from build123d import *

# Parameters (mm, degrees)
SKETCH1_W           = 25.4
SKETCH1_H           = 25.4
SKETCH1_W_2         = 22.225
SKETCH1_H_2         = 22.225
BOSS_EXTRUDE1_DEPTH = 330.2
SKETCH2_R           = 4.365625
SKETCH2_R_2         = 2.38125
CUT_EXTRUDE1_DEPTH  = 25.4


with BuildPart() as part:
    # Sketch1 → Boss-Extrude1 (new body)
    with BuildSketch(Plane(origin=(0, 0, 0), x_dir=(1, 0, 0), z_dir=(0, 1, 0))):
        Rectangle(SKETCH1_W, SKETCH1_H)
        Rectangle(SKETCH1_W_2, SKETCH1_H_2, mode=Mode.SUBTRACT)
    extrude(amount=BOSS_EXTRUDE1_DEPTH)

    # Sketch2 → Cut-Extrude1 (cut)
    with BuildSketch(Plane.XY.offset(12.7)):
        with Locations((0, 25.4)):
            Circle(SKETCH2_R)
        with Locations((0, 50.8)):
            Circle(SKETCH2_R)
        with Locations((0, 317.5)):
            Circle(SKETCH2_R_2)
        with Locations((0, 114.3)):
            Circle(SKETCH2_R_2)
    extrude(amount=-CUT_EXTRUDE1_DEPTH, mode=Mode.SUBTRACT)


solid = part.part
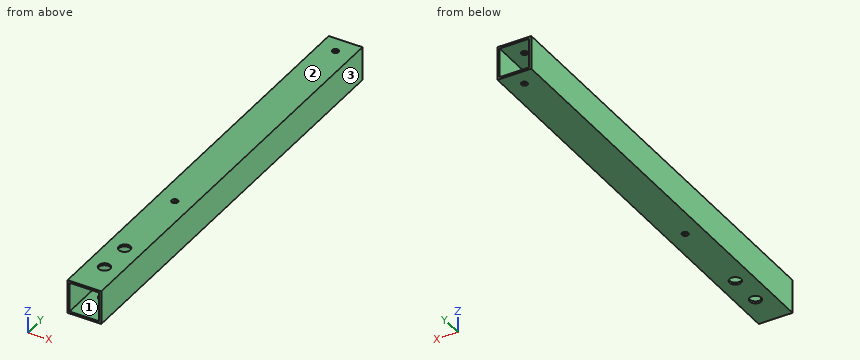
Verification items for the finished model (mm, model axes). Face numbers are marked on the shaded views. Give positions to 0.01 mm unless a question says otherwise; leave off trailing zeros. Loops run counter-clockwise (first coordinate to the right, second up) from the corner with the lowest first, then second, coordinate; pieces in that order, holes last. Notation, with made-up numbers: (-27, 74.25) - (20, 74.25) arc R19 ccw to (20, 98.25) - close; hole circle Ø4 at (53.5, 19.25). An arc over 180 degrees is marked (long way). Write item = value, one per line. Start each with the question number.
Q1. Cross-section at C-C, the plane y = 168. Enter the section's corners in (x, z).
Q2. Mould release check, pull along Z, two halves, no side actions. Record for the marked faces 1, 2 and 3: released by +Z, released by -Z, zero draft, split by the parting line, or undercut.
Q3. Cross-section at A-A, the plane z = 5. Enter the section's corners in (x, y), and give its area (3 significant figures).
Q4. Thickness scan on line 1 (Y direction, x = 0, z = 12.3); line 2 (X direction, y = 303, z = 5). Record the ranges inside material, lowest first.
Q5. Depth check by flat-ended pin: P1, Ø3, axis at x = 0, y = 317.5, coming from the +Z side. Enter the tip coordinate at first touch or a pass-through.
Q6. Cross-section at B-B, the plane y = 25.4. Enter the section's corners in (x, z), and give its area (3 significant figures).
Answer key:
q1.outline = (-12.7, -12.7) - (12.7, -12.7) - (12.7, 12.7) - (-12.7, 12.7) - close; hole (-11.11, -11.11) - (11.11, -11.11) - (11.11, 11.11) - (-11.11, 11.11) - close
q2.face_1 = undercut
q2.face_2 = released by +Z
q2.face_3 = zero draft
q3.outline = (-12.7, 0) - (-11.11, 0) - (-11.11, 330.2) - (-12.7, 330.2) - close; (11.11, 0) - (12.7, 0) - (12.7, 330.2) - (11.11, 330.2) - close
q3.area = 1,050 mm^2
q4.line_1 = 0 to 21.03, 29.77 to 46.43, 55.17 to 111.92, 116.68 to 315.12, 319.88 to 330.2
q4.line_2 = -12.7 to -11.11, 11.11 to 12.7
q5.P1 = through
q6.outline = (-12.7, -12.7) - (-4.37, -12.7) - (-4.37, -11.11) - (-11.11, -11.11) - (-11.11, 11.11) - (-4.37, 11.11) - (-4.37, 12.7) - (-12.7, 12.7) - close; (4.37, -12.7) - (12.7, -12.7) - (12.7, 12.7) - (4.37, 12.7) - (4.37, 11.11) - (11.11, 11.11) - (11.11, -11.11) - (4.37, -11.11) - close
q6.area = 123 mm^2
